Part print with two shaded views. Sizes in mm from the minimum x, y, z corner. Round coordinates to 2 decimals unless told otherwise and drop trailing zeros. Write each loop counter-clockwise with the first axis right and the second up, starting at its lowest first coordinate (ties: lowest second). Pieces come first, ordered by that corner, then holes. Notation, with made-up numbers: (-34, 8.25) -> (6, 8.25) arc R35 cw to (6, 45.25) -> close; hole circle Ø10 at (-17.75, 55.5). An arc over 180 degrees is marked (long way). Return JSON: item names as keys, results as strings.
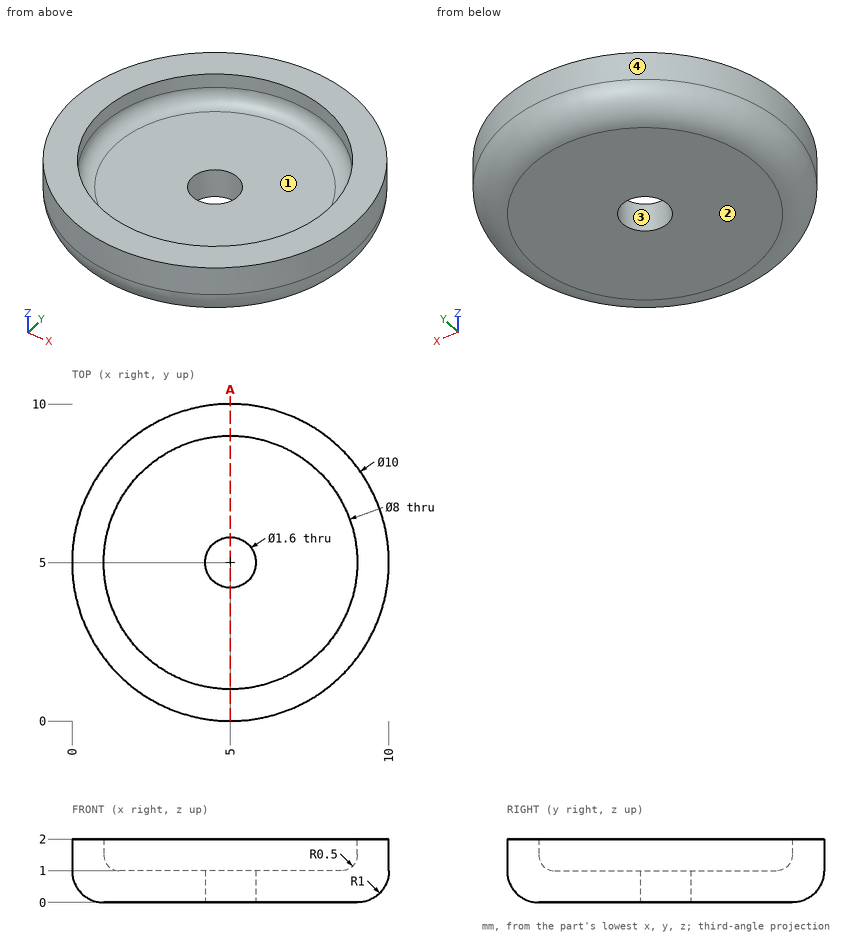
Q1. Pin check, flat tips, straight feed: pin 1 Ø1 at (x, y) = (7.5, 5.5) entering from +Z; pin 2 Ø1 at (y, z) = (7, 0.5) entering from -X. Stop position of each tip, or through.
Verdict:
{"pin 1": "stops at z = 1", "pin 2": "stops at x = 0.28"}
Q2. Two-plate mould, pull along Y, no slides. Class the marked faces 1, 2, 3 and 4: +Y half, -Y half, draft (parallel to the pull), parting line (faces both ways), or undercut.
Verdict:
{"face 1": "undercut", "face 2": "draft", "face 3": "undercut", "face 4": "parting line"}
Q3. Wall check: L1, parallel to Y at x = 5, z = 1.85; L2, parallel to Y at x = 8, z = 1.85; L3, parallel to Z at x = 7.75, y = 3. Give the ranges that are in metal, low to high.
Verdict:
{"L1": "y = 0 to 1, 9 to 10", "L2": "y = 1 to 2.35, 7.65 to 9", "L3": "z = 0 to 1"}
Q4. Saw through at A-A on x = 5. List the corners of the cut face in (y, z).
Verdict:
{"outline": "(0, 1) arc R1 ccw to (1, 0) -> (4.2, 0) -> (4.2, 1) -> (1.5, 1) arc R0.5 cw to (1, 1.5) -> (1, 2) -> (0, 2) -> close; (5.8, 0) -> (9, 0) arc R1 ccw to (10, 1) -> (10, 2) -> (9, 2) -> (9, 1.5) arc R0.5 cw to (8.5, 1) -> (5.8, 1) -> close"}
